Model file for the job. Use its own axes, mm. Face numbers are marked on the shaded views. Coordinates: 2 decimals unless noted, no trailing zeros. Loops run counter-clockwise (first coordinate to the right, second up) from the corner with the lowest first, then second, coordinate; pieces in that order, holes last.
from build123d import *

# Parameters (mm, degrees)
F0_R     = 17.5
F1_DEPTH = 1


with BuildPart() as f1:
    # F0 (on Top) → F1 (new body)
    with BuildSketch(Plane.XY):
        with BuildLine():
            ThreePointArc((-74.232287, -10.703622), (-49.103097, -56.691144), (0, -75))
            Line((0, -75), (0, -66.83293))
            ThreePointArc((0, -66.83293), (-43.756051, -50.517803), (-66.148816, -9.538059))
            Line((-66.148816, -9.538059), (-74.232287, -10.703622))
        make_face()
        with BuildLine():
            Line((66.148816, 9.538059), (74.232287, 10.703622))
            ThreePointArc((74.232287, 10.703622), (49.103097, 56.691144), (0, 75))
            Line((0, 75), (0, 66.83293))
            ThreePointArc((0, 66.83293), (43.756051, 50.517803), (66.148816, 9.538059))
        make_face()
        with BuildLine():
            ThreePointArc((66.83293, 0), (66.661682, 4.781281), (66.148816, 9.538059))
            ThreePointArc((66.148816, 9.538059), (43.756051, 50.517803), (0, 66.83293))
            ThreePointArc((0, 66.83293), (-50.517803, 43.756051), (-66.148816, -9.538059))
            ThreePointArc((-66.148816, -9.538059), (-43.756051, -50.517803), (0, -66.83293))
            ThreePointArc((0, -66.83293), (47.258018, -47.258018), (66.83293, 0))
        make_face()
        Circle(F0_R, mode=Mode.SUBTRACT)
    extrude(amount=F1_DEPTH)


solid = f1.part
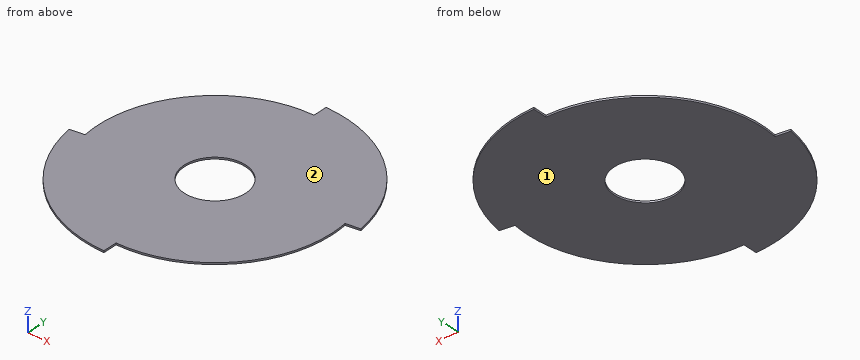
Q1. Drill centre lines: line 1 (Y direction, x = 9, z = 0.65); line 2 (X direction, y = 53, z = 0.75); line 3 (X direction, y = 60, z = 0.5). Where is each one in solid material? Low to high.
Answers:
line 1: y = -66.22 to -15.01, 15.01 to 74.46
line 2: x = -40.71 to 53.07
line 3: x = -29.44 to 45
Q2. Slice it at C-C (y = 15). List the corners of the cut face in (x, z).
Answers:
outline: (-65.13, 0) - (-9.01, 0) - (-9.01, 1) - (-65.13, 1) - close; (9.01, 0) - (73.48, 0) - (73.48, 1) - (9.01, 1) - close
Q3. Mould opens along Z. For the marked faces 1 and 2 say: +Z half, -Z half, draft (parallel to the pull), parting line (faces both ways), or undercut.
Answers:
face 1: -Z half
face 2: +Z half
Q4. Slice it at B-B (x = 6.5). List the corners of the cut face in (y, z).
Answers:
outline: (-66.52, 0) - (-16.25, 0) - (-16.25, 1) - (-66.52, 1) - close; (16.25, 0) - (74.72, 0) - (74.72, 1) - (16.25, 1) - close
Q5. Slice it at D-D (y = 46.5). List the corners of the cut face in (x, z).
Answers:
outline: (-48, 0) - (58.85, 0) - (58.85, 1) - (-48, 1) - close
Q6. Slice it at A-A (z = 0.3). List the corners of the cut face in (x, y).
Answers:
outline: (-74.23, -10.7) arc R75 ccw to (0, -75) - (0, -66.83) arc R66.83 ccw to (66.83, 0) arc R66.83 ccw to (66.15, 9.54) - (74.23, 10.7) arc R75 ccw to (0, 75) - (0, 66.83) arc R66.83 ccw to (-66.15, -9.54) - close; hole circle Ø35 at (0, 0)
